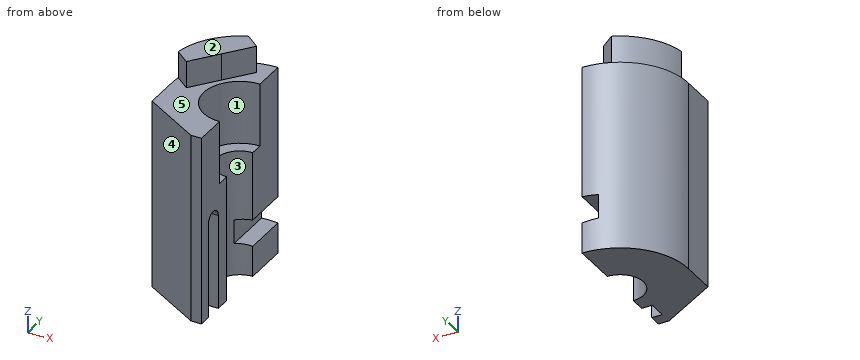
```python
from build123d import *

# Parameters (mm, degrees)
BOSS_EXTRUDE1_DEPTH     = 234
SKETCH2_R               = 44.45
CUT_EXTRUDE2_DEPTH      = 78
SKETCH3_R               = 28.575
CUT_EXTRUDE3_DEPTH      = 301.059994001
CUT_EXTRUDE4_DEPTH      = 13
BOSS_EXTRUDE2_START     = 33
BOSS_EXTRUDE2_DEPTH     = 33
CUT_EXTRUDE6_REACH      = 302.06
CUT_EXTRUDE6_END_RADIUS = 28.575


with BuildPart() as part:
    # Sketch1 → Boss-Extrude1 (new body)
    with BuildSketch(Plane.XY):
        with BuildLine():
            Line((0, 0), (-13, 0))
            Line((-13, 0), (-84, 40.991869112))
            Line((-84, 40.991869112), (-84, 84))
            ThreePointArc((-84, 84), (-59.39696962, 143.39696962), (0, 168))
            Line((0, 168), (0, 0))
        make_face()
    extrude(amount=-BOSS_EXTRUDE1_DEPTH)

    # Sketch2 → Cut-Extrude2 (cut)
    with BuildSketch(Plane.XY):
        with Locations((0, 84)):
            Circle(SKETCH2_R)
    extrude(amount=-CUT_EXTRUDE2_DEPTH, mode=Mode.SUBTRACT)

    # Sketch3 → Cut-Extrude3 (cut, through all)
    with BuildSketch(Plane.XY):
        with Locations((0, 84)):
            Circle(SKETCH3_R)
    extrude(amount=-CUT_EXTRUDE3_DEPTH, mode=Mode.SUBTRACT)

    # Sketch5 → Cut-Extrude4 (cut)
    with BuildSketch(Plane(origin=(0, 0, 0), x_dir=(0, 0, -1), z_dir=(1, 0, 0))):
        with BuildLine():
            Line((234, 15), (117, 15))
            ThreePointArc((117, 15), (106, 26), (117, 37))
            Line((117, 37), (234, 37))
            ThreePointArc((234, 37), (245, 26), (234, 15))
        make_face()
    extrude(amount=-CUT_EXTRUDE4_DEPTH, mode=Mode.SUBTRACT)

    # Sketch6 → Boss-Extrude2 (add)
    with BuildSketch(Plane.XY.offset(BOSS_EXTRUDE2_START)):
        with BuildLine():
            Line((-40.188548434, 115.398735242), (-14.946427946, 147.707176139))
            Line((-14.946427946, 147.707176139), (-32.530408402, 161.445287327))
            ThreePointArc((-32.530408402, 161.445287327), (-66.192903303, 135.715563927), (-83.014649379, 96.828405531))
            Line((-83.014649379, 96.828405531), (-65.430668922, 83.090294344))
            Line((-65.430668922, 83.090294344), (-40.188548434, 115.398735242))
        make_face()
    extrude(amount=-BOSS_EXTRUDE2_DEPTH)

    # Cut-Extrude6: up to this cylinder (the profile starts outside it)
    cut_extrude6_end = Plane(origin=(0, 84, -179.5), z_dir=(0, 0, 1)) * Cylinder(CUT_EXTRUDE6_END_RADIUS, 662.27, mode=Mode.PRIVATE)
    # Sketch7 → Cut-Extrude6 (cut, up to the surface)
    with BuildSketch(Plane(origin=(0, 168, 0), x_dir=(1, 0, 0), z_dir=(0, 1, 0)), mode=Mode.PRIVATE) as cut_extrude6_sk1:
        Polygon((0, 196), (-19, 194.337715393), (-19, 164.662284607), (0, 163), align=None)
    cut_extrude6_tool1 = extrude(cut_extrude6_sk1.sketch, amount=-CUT_EXTRUDE6_REACH, mode=Mode.PRIVATE) - cut_extrude6_end
    add(cut_extrude6_tool1.solids().sort_by_distance((-9.332027, 168, -179.5))[0], mode=Mode.SUBTRACT)


solid = part.part
```
Input: part model. Units: mm. Frame: model coordinates. Face numbers are marked on the shaded views. A direction names the side the tool comes from. Coordinates: 2 decimals unless noted, no trailing zeros. Order: outer loops, then holes, each group sorted by start corner. A loop starts at its lowest first (then second) coordinate and runs counter-clockwise, first axis right, second up. Notation, with made-up numbers: (24, 1.25) - (45, 1.25) arc R12 ccw to (45, 8.25) - close; hole circle Ø6 at (-16.75, 18.25). An arc over 180 degrees is marked (long way). Put each result on its own line as item: value.
1. Cut plane D-D on z = -84. Return the cut outline in (x, y) (3 decimals).
Report:
outline: (-84, 40.992) - (-13, 0) - (0, 0) - (0, 55.425) arc R28.575 cw to (0, 112.575) - (0, 168) arc R84 ccw to (-84, 84) - close
2. Draft query along Y for the marked faces 3, 4 and 5. Return one class per face: pulls with the +Y half, pulls with the -Y half, needs draft (parallel to the pull), parting line crosses it, or undercut.
Report:
face 3: undercut
face 4: pulls with the -Y half
face 5: needs draft
3. Cut plane C-C on y = 93. Return the cut outline in (x, z), then the cut area to 3 significant figures.
Report:
outline: (-83.52, -234) - (-27.12, -234) - (-27.12, -78) - (-43.53, -78) - (-43.53, 0) - (-57.69, 0) - (-57.69, 33) - (-78.11, 33) - (-78.11, 0) - (-83.52, 0) - close
area: 12,600 mm2
4. Reachability of the marked faces 1 and 2 from +Z, -Z, +X, -X, +Y, -Y: full face, straight path, thin tool, end or side. Return the list, or none.
Report:
face 1: +Z, +X
face 2: +Z, +X, -X, +Y, -Y
5. Line query: line 1 along Z through (x, y) = (-65.5, 59.5); line 2 along Y through (x, z) = (-24, -25.5); line 3 along Y through (x, z) = (-19.5, -197.5). Output: solid intervals per line, ascending.
Report:
line 1: z = -234 to 0
line 2: y = 6.35 to 46.59, 121.41 to 164.5
line 3: y = 3.75 to 63.11, 104.89 to 165.71
6. Cut plane B-B on x = -54.5. Return the cut outline in (y, z), then the cut area to 3 significant figures.
Report:
outline: (23.96, -234) - (147.92, -234) - (147.92, 33) - (97.08, 33) - (97.08, 0) - (23.96, 0) - close
area: 30,700 mm2
7. Cut plane A-A on z = -159. Return the cut outline in (x, y) (3 decimals).
Report:
outline: (-84, 40.992) - (-13, 0) - (0, 0) - (0, 15) - (-13, 15) - (-13, 37) - (0, 37) - (0, 55.425) arc R28.575 cw to (0, 112.575) - (0, 168) arc R84 ccw to (-84, 84) - close
8. Contact query for flat-ended pins moving along their axis: pin 1 Ø1.5 at (x, z) = (-71, -84.5) entering from -Y; pin 2 Ø17.5 at (y, z) = (22.5, -198) entering from +X; pin 3 Ø10 at (y, z) = (69.5, -49) entering from +X; pin 4 Ø13.5 at (x, y) = (-32, 89) entering from +Z. Output: stop coordinate, or through.
Report:
pin 1: stops at y = 33.05
pin 2: stops at x = 0
pin 3: stops at x = -39.94
pin 4: stops at z = -78
